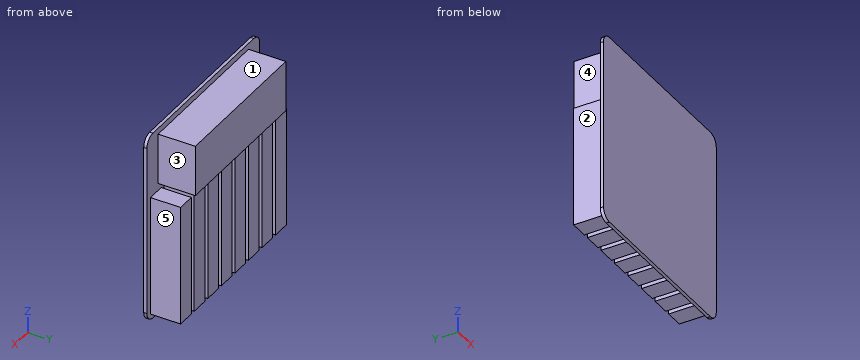
from build123d import *

# Parameters (mm, degrees)
SKETCH1_W           = 95
SKETCH1_H           = 95
BOSS_EXTRUDE1_DEPTH = 0.8
FILLET1_R           = 5
SKETCH2_W           = 76.2
SKETCH2_H           = 25.4
BOSS_EXTRUDE2_DEPTH = 18.542
SKETCH3_W           = 9
SKETCH3_H           = 60
BOSS_EXTRUDE3_DEPTH = 15


with BuildPart() as part:
    # Sketch1 → Boss-Extrude1 (new, symmetric)
    with BuildSketch(Plane(origin=(0, 0, 0), x_dir=(1, 0, 0), z_dir=(0, 1, 0))):
        Rectangle(SKETCH1_W, SKETCH1_H)
    extrude(amount=BOSS_EXTRUDE1_DEPTH, both=True)

    # Fillet1
    fillet1_edges = [part.edges().sort_by_distance(p)[0] for p in [
        (47.5, 0, 47.5),
        (-47.5, 0, 47.5),
        (-47.5, 0, -47.5),
        (47.5, 0, -47.5),
    ]]
    fillet(fillet1_edges, radius=FILLET1_R)

    # Sketch2 → Boss-Extrude2 (add)
    with BuildSketch(Plane(origin=(0, 0.8, 0), x_dir=(1, 0, 0), z_dir=(0, 1, 0))):
        with Locations((0, -31.8)):
            Rectangle(SKETCH2_W, SKETCH2_H)
    extrude(amount=BOSS_EXTRUDE2_DEPTH)

    # Sketch3 → Boss-Extrude3 (add)
    with BuildSketch(Plane(origin=(0, 0.8, 0), x_dir=(1, 0, 0), z_dir=(0, 1, 0))):
        with Locations((-40, 14.5)):
            Rectangle(SKETCH3_W, SKETCH3_H)
        with Locations((-28.571428571, 14.5)):
            Rectangle(SKETCH3_W, SKETCH3_H)
        with Locations((-17.142857143, 14.5)):
            Rectangle(SKETCH3_W, SKETCH3_H)
        with Locations((-5.714285714, 14.5)):
            Rectangle(SKETCH3_W, SKETCH3_H)
        with Locations((5.714285714, 14.5)):
            Rectangle(SKETCH3_W, SKETCH3_H)
        with Locations((17.142857143, 14.5)):
            Rectangle(SKETCH3_W, SKETCH3_H)
        with Locations((28.571428571, 14.5)):
            Rectangle(SKETCH3_W, SKETCH3_H)
        with Locations((40, 14.5)):
            Rectangle(SKETCH3_W, SKETCH3_H)
    extrude(amount=BOSS_EXTRUDE3_DEPTH)


solid = part.part
Here's how the part is built. I have some questions about the finished solid (model axes, mm). Face numbers are marked on the shaded views. A direction names the side the tool comes from. Coordinates: 2 decimals unless noted, no trailing zeros. Write each loop counter-clockwise with the first axis right and the second up, starting at its lowest first coordinate (ties: lowest second). Pieces come first, ordered by that corner, then holes.
Item 1: If I drill on line 1 (Z direction, x = -14.5, y = 14.75); line 2 (X direction, y = 9.25, z = 22.5); line 3 (Y direction, x = 5, z = -5.5), over which ranges is the centre line in solid material (lowest first)?
Item 2: On a 3-axis mill with a long thin cutter (end or side, diameter ignored), from which of +Z, -Z, +X, -X, +Y, -Y can I reach the whole of each face in a straight line? I mean the marked faces 1, 2, 3, 4 and 5. Say none if no direction works.
Item 3: I want a section at C-C on y = 5. Count the separate pieces of the cut face and the enclosed holes in it, and give its area (3 significant figures).
Item 4: Will these pins go through, and if not, where does the flat tip stop? pin 1 (4 mm diameter, centred on y = 14.5, z = -10.5, fed in from -X); pin 2 (6 mm diameter, centred on x = 18.5, z = -25.5, fed in from +Y); pin 3 (10 mm diameter, centred on x = 19, y = 8, fed in from +Z); pin 4 (4 mm diameter, centred on y = 1.5, z = 34.5, fed in from +X).
Item 5: I want a section at B-B on z = 41. Write out the boundary of the cut face in (x, y), and give its area (3 significant figures).
Item 6: I want a section at A-A on x = 37. Write out the boundary of the cut face in (y, z), and give its area (3 significant figures).
Findings below:
1. line 1: z = -44.5 to 15.5, 19.1 to 44.5
1. line 2: x = -38.1 to 38.1
1. line 3: y = -0.8 to 15.8
2. face 1: +Z, +X, -X, +Y
2. face 2: +Z, -Z, -X, +Y
2. face 3: +Z, +X, +Y
2. face 4: +Z, -X, +Y
2. face 5: +Z, -Z, +X, +Y
3. separate pieces: 9
3. enclosed holes: 0
3. area: 6,260 mm2
4. pin 1: stops at x = -44.5
4. pin 2: stops at y = 15.8
4. pin 3: stops at z = 44.5
4. pin 4: stops at x = 47.5
5. outline: (-47.5, -0.8) - (47.5, -0.8) - (47.5, 0.8) - (38.1, 0.8) - (38.1, 19.34) - (-38.1, 19.34) - (-38.1, 0.8) - (-47.5, 0.8) - close
5. area: 1,560 mm2
6. outline: (-0.8, -47.5) - (0.8, -47.5) - (0.8, -44.5) - (15.8, -44.5) - (15.8, 15.5) - (0.8, 15.5) - (0.8, 19.1) - (19.34, 19.1) - (19.34, 44.5) - (0.8, 44.5) - (0.8, 47.5) - (-0.8, 47.5) - close
6. area: 1,520 mm2
